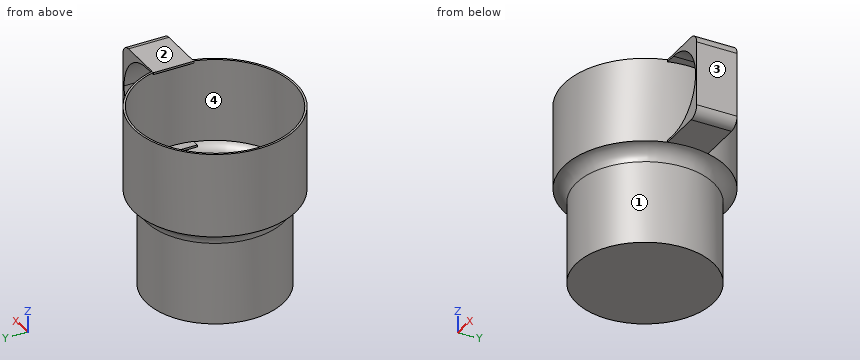
from build123d import *

# Parameters (mm, degrees)
F2_T     = -1
F4_DEPTH = 10


with BuildPart() as f1:
    # F0 (on Front) → F1 (revolve)
    with BuildSketch(Plane.XZ):
        with BuildLine():
            Line((-34, 0), (0, 0))
            Line((0, 0), (0, 90))
            Line((0, 90), (-40, 90))
            Line((-40, 90), (-40, 48))
            ThreePointArc((-40, 48), (-35.706514, 45.627105), (-34, 41.027925))
            Line((-34, 41.027925), (-34, 0))
        make_face()
    revolve(axis=Axis((0, 0, 45), (0, 0, 1)))

    # F2
    f2_openings = [f1.faces().sort_by_distance(p)[0] for p in [
        (0, 0, 90),
    ]]
    offset(amount=F2_T, openings=f2_openings)

    # F3 (on Front) → F4 (join, symmetric)
    with BuildSketch(Plane.XZ):
        with BuildLine():
            Line((60, 90), (37.403014, 90))
            Line((37.403014, 90), (37.403014, 89))
            Line((37.403014, 89), (44, 89))
            ThreePointArc((44, 89), (58.142136, 83.142136), (64, 69))
            ThreePointArc((64, 69), (58.142136, 54.857864), (44, 49))
            Line((44, 49), (34.291856, 49))
            Line((34.291856, 49), (34.291856, 48))
            Line((34.291856, 48), (60, 48))
            ThreePointArc((60, 48), (63.535534, 49.464466), (65, 53))
            Line((65, 53), (65, 85))
            ThreePointArc((65, 85), (63.535534, 88.535534), (60, 90))
        make_face()
    extrude(amount=F4_DEPTH, both=True)


solid = f1.part
Here's how the part is built. I have some questions about the finished solid (model axes, mm). Face numbers are marked on the shaded views. Round coordinates to 2 decimals unless told otherwise and drop trailing zeros. Loops run counter-clockwise (first coordinate to the right, second up) from the corner with the lowest first, then second, coordinate; pieces in that order, holes last. Notation, with made-up numbers: (62, -15) - (106, -15) arc R17 cw to (106, -11) - close; hole circle Ø7 at (-17, 18). An arc over 180 degrees is marked (long way). One line per question, with ' | ' between items. Start each with the question number.
Q1. I want a section at D-D (z = 37.5). Write out the boundary of the cut face in (x, y), then the cut area to 3 significant figures.
Q2. We'd pull the mould along X, two halves only. Please class the marked faces 1, 2, 3 and 4: +X half, -X half, draft (parallel to the pull), parting line (faces both ways), or undercut.
Q3. I want a section at C-C (x = 0). Write out the boundary of the cut face in (y, z), then the cut area to 3 significant figures.
Q4. Please list where these lines run through material, in increasing order: line 1 (Y direction, x = 0, z = 32); line 2 (Y direction, x = 0, z = 67). Write a range as [from, to].
Q5. I want a section at B-B (x = 48.5). Write out the boundary of the cut face in (y, z).
Q6. Will these pins go through, and if not, where does the flat tip stop? pin 1 (1.1 mm diameter, centred on y = -4.5, z = 48.5, fed in from -X); pin 2 (2 mm diameter, centred on y = -19.5, z = 61.5, fed in from -X); pin 3 (1.3 mm diameter, centred on x = 38, y = 2.5, fed in from -Z).
Response values:
1) outline: circle Ø68 at (0, 0); hole circle Ø66 at (0, 0) | area: 210 mm²
2) face 1: parting line | face 2: draft | face 3: +X half | face 4: undercut
3) outline: (-40, 48) arc R7.05 cw to (-34, 41.03) - (-34, 0) - (34, 0) - (34, 41.03) arc R7.05 cw to (40, 48) - (40, 90) - (39, 90) - (39, 48.81) arc R8.05 ccw to (33, 41.03) - (33, 1) - (-33, 1) - (-33, 41.03) arc R8.05 ccw to (-39, 48.81) - (-39, 90) - (-40, 90) - close | area: 252 mm²
4) line 1: y = [-34, -33], [33, 34] | line 2: y = [-40, -39], [39, 40]
5) outline: (-10, 48) - (10, 48) - (10, 49.51) - (-10, 49.51) - close; (-10, 88.49) - (10, 88.49) - (10, 90) - (-10, 90) - close
6) pin 1: stops at x = -39.8 | pin 2: stops at x = -35.46 | pin 3: stops at z = 47.08
